from build123d import *

# Parameters (mm, degrees)
SKETCH1_R           = 59.910502434
BOSS_EXTRUDE1_DEPTH = 44.958
SKETCH2_R           = 30.133554255
BOSS_EXTRUDE2_DEPTH = 177.8
SKETCH3_W           = 54.540648196
SKETCH3_H           = 11.308105597
SKETCH3_H_2         = 15.077164852
CUT_EXTRUDE4_DEPTH  = 76.2
SKETCH5_R           = 12.7
CUT_EXTRUDE5_DEPTH  = 85.390003891


with BuildPart() as part:
    # Sketch1 → Boss-Extrude1 (new body)
    with BuildSketch(Plane(origin=(0, 0, 0), x_dir=(1, 0, 0), z_dir=(0, 1, 0))):
        Circle(SKETCH1_R)
    extrude(amount=BOSS_EXTRUDE1_DEPTH)

    # Sketch2 → Boss-Extrude2 (add)
    with BuildSketch(Plane(origin=(0, 44.958, 0), x_dir=(1, 0, 0), z_dir=(0, 1, 0))):
        Circle(SKETCH2_R)
    extrude(amount=BOSS_EXTRUDE2_DEPTH)

    # Sketch3 → Cut-Extrude4 (cut)
    with BuildSketch(Plane(origin=(0, 222.758, 0), x_dir=(1, 0, 0), z_dir=(0, 1, 0))):
        with Locations((0, 30.133554255)):
            Rectangle(SKETCH3_W, SKETCH3_H)
        with Locations((0, -30.133554255)):
            Rectangle(SKETCH3_W, SKETCH3_H_2)
    extrude(amount=-CUT_EXTRUDE4_DEPTH, mode=Mode.SUBTRACT)

    # Sketch5 → Cut-Extrude5 (cut, through all)
    with BuildSketch(Plane(origin=(0, 0, -24.479501456), x_dir=(-1, 0, 0), z_dir=(0, 0, -1))):
        with Locations((0, 197.652270739)):
            Circle(SKETCH5_R)
    extrude(amount=-CUT_EXTRUDE5_DEPTH, mode=Mode.SUBTRACT)


solid = part.part
Geometry: final body of the model. Coordinates: model frame, mm. A direction names the side the tool comes from. Give positions to 0.01 mm unless a question says otherwise; leave off trailing zeros. Order: outer loops, then holes, each group sorted by start corner. A loop starts at its lowest first (then second) coordinate and runs counter-clockwise, first axis right, second up. Notation, with made-up numbers: (-12.75, 35.25) -> (46.25, 35.25) arc R18 ccw to (46.25, 58.25) -> close; hole circle Ø2 at (-34.5, 68.5). An arc over 180 degrees is marked (long way). Answer as a JSON object with one key per item and string values.
Q1. First-contact query: pin 1 (1.5 mm diameter, centred on y = 57, z = -23.5, fed in from -X); pin 2 (10.5 mm diameter, centred on x = -2.5, y = 175, fed in from -Z); pin 3 (12 mm diameter, centred on x = -28, y = 153, fed in from +Z); pin 4 (12 mm diameter, centred on x = -3.5, y = 197.5, fed in from +Z). Flat tips, straight axial feed; report the tip coordinate or a pass-through.
Entries:
{"pin 1": "stops at x = -19.76", "pin 2": "stops at z = -24.48", "pin 3": "stops at z = 20.59", "pin 4": "passes through"}
Q2. Material intervals for probe 1 along Y at (x, z) = (0, 8); probe 2 along Y at (x, z) = (52, 23); probe 3 along Z at (x, y) = (0, 140), sorted ascending.
Entries:
{"probe 1": "y = 0 to 184.95, 210.35 to 222.76", "probe 2": "y = 0 to 44.96", "probe 3": "z = -30.13 to 30.13"}
Q3. Access query for faces 4 (the cylindrical face through (-12.987, 22.164, 58.486)), 5 (the flat face through (4, 185, 22.595)), 6 (the flat face through (-27, 44.958, -14)), 7 (the flat face through (-4, 185, -24.48)). Directions: +Z, -Z, +X, -X, +Y, -Y. A direction counts if a zero-diameter tool reaches every point of the face in a straight line with its end or side. Return the directions, or none.
Entries:
{"face 4": "+Y, -Y", "face 5": "+Z, +X, -X, +Y", "face 6": "+Y", "face 7": "-Z, +X, -X, +Y"}
Q4. Section C-C (y = 189). Output: boundary loops of the cut face in (x, z).
Entries:
{"outline": "(-19.94, 22.59) arc R30.13 ccw to (-17.57, -24.48) -> (-9.3, -24.48) -> (-9.3, 22.59) -> close; (9.3, -24.48) -> (17.57, -24.48) arc R30.13 ccw to (19.94, 22.59) -> (9.3, 22.59) -> close"}
Q5. Section D-D (x = -23). Output: boundary loops of the cut face in (y, z).
Entries:
{"outline": "(0, -55.32) -> (44.96, -55.32) -> (44.96, -19.47) -> (222.76, -19.47) -> (222.76, 19.47) -> (44.96, 19.47) -> (44.96, 55.32) -> (0, 55.32) -> close"}
Q6. Section B-B (z = 0). Output: boundary loops of the cut face in (x, y).
Entries:
{"outline": "(-59.91, 0) -> (59.91, 0) -> (59.91, 44.96) -> (30.13, 44.96) -> (30.13, 222.76) -> (-30.13, 222.76) -> (-30.13, 44.96) -> (-59.91, 44.96) -> close; hole circle Ø25.4 at (0, 197.65)"}
Q7. Draft query along Y for faces 1 (the cylindrical face through (2.753, 185.254, -1.272)), 2 (the cylindrical face through (-30.104, 112.858, -1.325)), 3 (the flat face through (0, 146.558, -27)). Return one class per face: released by +Y, released by -Y, zero draft, split by the parting line, or undercut.
Entries:
{"face 1": "undercut", "face 2": "zero draft", "face 3": "released by +Y"}
Q8. Section A-A (x = 0). Output: boundary loops of the cut face in (y, z).
Entries:
{"outline": "(0, -59.91) -> (44.96, -59.91) -> (44.96, -30.13) -> (146.56, -30.13) -> (146.56, -24.48) -> (184.95, -24.48) -> (184.95, 22.59) -> (146.56, 22.59) -> (146.56, 30.13) -> (44.96, 30.13) -> (44.96, 59.91) -> (0, 59.91) -> close; (210.35, -24.48) -> (222.76, -24.48) -> (222.76, 22.59) -> (210.35, 22.59) -> close"}
